Read the model definition and answer for the solid it produces. Units are mm, in the model's axes. Coordinates: 2 decimals unless noted, no trailing zeros. Write each loop counter-clockwise with the first axis right and the second up, starting at its lowest first coordinate (ties: lowest second). Pieces come first, ordered by that corner, then holes.
1) The part is cut by section A-A (y = 0). Determine the outline of the cut face in (x, z).
2) Find the intervals of material crossed by line 1 (Y direction, x = -18, z = 1.5); line 2 (Y direction, x = -14, z = 3); line 3 (Y direction, x = 31, z = 3.95), in increasing order.
3) The part is cut by section B-B (x = 31). Determine the outline of the cut face in (y, z).
4) Each of these flat-tipped pins is pushed along its axis until it touches: pin 1 Ø1 at (y, z) = (4, 2.5) entering from -X; pin 2 Ø2 at (y, z) = (-15, 1) entering from +X; pin 3 Ø5 at (x, y) = (-15.5, -26.85) entering from +Z; pin 4 Ø7.5 at (x, y) = (15.5, 26.85) entering from -Z. Where does it stop, or does it pass through?
5) Determine the mould class of faces 1 (the face through (-1, 1, 0)), 2 (the face through (-33.875, 0.378, 3.783)), 3 (the face through (17.535, 33.713, 2.465)) for opening direction X: +X half, -X half, draft (parallel to the pull), parting line (faces both ways), or undercut.
6) The part is cut by section C-C (x = -15.5). Determine the outline of the cut face in (y, z), then the cut area to 3 significant figures.
Solid Edge part; units mm, degrees
sketch "Sketch1" plane through (0, 0, 0) normal (0, 0, 1) x (1, 0, 0)
  circle A0 centre (0, 0) radius 38
extrude "Protrusion1" add sketch "Sketch1" along normal blind 5
hole "Hole_1" at (31, 0, 0) direction (0, 0, 1) diameter 5.8 end up to next countersink diameter 11 countersink angle 90
pattern_circular "Pattern1" count 6 over 360 about axis through (0, 0, 0) along (0, 0, 1) of "Hole_1"
properties material "Steel"
Reported:
1. outline: (-38, 0) - (-36.5, 0) - (-33.9, 2.6) - (-33.9, 5) - (-38, 5) - close; (-28.1, 2.6) - (-25.5, 0) - (25.5, 0) - (28.1, 2.6) - (28.1, 5) - (-28.1, 5) - close; (33.9, 2.6) - (36.5, 0) - (38, 0) - (38, 5) - (33.9, 5) - close
2. line 1: y = -33.47 to -29.97, -23.72 to 23.72, 29.97 to 33.47
2. line 2: y = -35.33 to -29.33, -24.36 to 24.36, 29.33 to 35.33
2. line 3: y = -21.98 to -2.9, 2.9 to 21.98
3. outline: (-21.98, 0) - (-5.5, 0) - (-2.9, 2.6) - (-2.9, 5) - (-21.98, 5) - close; (2.9, 2.6) - (5.5, 0) - (21.98, 0) - (21.98, 5) - (2.9, 5) - close
4. pin 1: stops at x = -37.84
4. pin 2: stops at x = 35.33
4. pin 3: passes through
4. pin 4: stops at z = 1.75
5. face 1: draft
5. face 2: undercut
5. face 3: parting line
6. outline: (-34.7, 0) - (-32.35, 0) - (-29.75, 2.6) - (-29.75, 5) - (-34.7, 5) - close; (-23.95, 2.6) - (-21.35, 0) - (21.35, 0) - (23.95, 2.6) - (23.95, 5) - (-23.95, 5) - close; (29.75, 2.6) - (32.35, 0) - (34.7, 0) - (34.7, 5) - (29.75, 5) - close
6. area: 275 mm2
